Model file for the job. Use its own axes, mm. A direction names the side the tool comes from. Round coordinates to 2 decimals unless told otherwise and drop trailing zeros. Loops run counter-clockwise (first coordinate to the right, second up) from the corner with the lowest first, then second, coordinate; pieces in that order, holes last. Notation, with made-up numbers: (51.25, 43.25) -> (77.25, 43.25) arc R15 ccw to (77.25, 67.25) -> close; hole circle Ø5 at (22.25, 43.5). An arc over 180 degrees is marked (long way). Use a Markdown table: item, result. Add a question column.
```python
from build123d import *

# Parameters (mm, degrees)
SKETCH1_R           = 22.5
BOSS_EXTRUDE3_DEPTH = 20
SKETCH4_R           = 21
CUT_EXTRUDE2_DEPTH  = 10
SKETCH5_R           = 15
BOSS_EXTRUDE4_DEPTH = 20
SKETCH6_R           = 10
CUT_EXTRUDE4_DEPTH  = 20


with BuildPart() as part:
    # Sketch1 → Boss-Extrude3 (new body)
    with BuildSketch(Plane.XY):
        Circle(SKETCH1_R)
    extrude(amount=BOSS_EXTRUDE3_DEPTH)

    # Sketch4 → Cut-Extrude2 (cut)
    with BuildSketch(Plane.XY.offset(20)):
        Circle(SKETCH4_R)
    extrude(amount=-CUT_EXTRUDE2_DEPTH, mode=Mode.SUBTRACT)

    # Sketch5 → Boss-Extrude4 (add)
    with BuildSketch(Plane(origin=(0, 0, 0), x_dir=(-1, 0, 0), z_dir=(0, 0, -1))):
        Circle(SKETCH5_R)
    extrude(amount=BOSS_EXTRUDE4_DEPTH)

    # Sketch6 → Cut-Extrude4 (cut)
    with BuildSketch(Plane(origin=(0, 0, -20), x_dir=(-1, 0, 0), z_dir=(0, 0, -1))):
        Circle(SKETCH6_R)
    extrude(amount=-CUT_EXTRUDE4_DEPTH, mode=Mode.SUBTRACT)


solid = part.part
```
1) Cut at C-C on y = 17.5. Write the cut outline in (x, z), and give its area (3 significant figures).
2) Tool access for faces 4 (the face through (10.382, -19.961, 9.86)), 5 (the face through (0, 0, 10)), 6 (the face through (2.17, -9.76, -10.14)): list every direction of +Z, -Z, +X, -X, +Y, -Y with a clear straight run to the whole face (end or side of a thin tool).
3) Pin check, flat tips, straight feed: pin 1 Ø1 at (x, z) = (2.5, 14.5) entering from +Y; pin 2 Ø12.5 at (x, y) = (6, 9) entering from +Z; pin 3 Ø18 at (x, y) = (0, 0) entering from -Z; pin 4 Ø1.5 at (y, z) = (17, -14) entering from -X. Stop position of each tip, or through.
4) Cut at A-A on y = 0. Write the cut outline in (x, z), and give its area (3 significant figures).
5) Wall check: probe 1 along Y at (x, z) = (0, 14); probe 2 along Y at (x, z) = (0, -11.5); probe 3 along Z at (x, y) = (2, -1). Give the ranges that are in metal, low to high. Write a range as from..to.
6) Pull direction X, two halves, no side cores. Call faces 1 (the face through (-3, -10, -20)), 2 (the face through (14.985, 0.66, -9.86)), 3 (the face through (20.03, 6.31, 15.07)): +X half, -X half, draft (parallel to the pull), parting line (faces both ways), or undercut.
7) Cut at B-B on x = 18.5. Write the cut outline in (y, z), and give its area (3 significant figures).
Established:
| question | item | result |
|---|---|---|
| 1 | outline | (-14.14, 0) -> (14.14, 0) -> (14.14, 20) -> (11.61, 20) -> (11.61, 10) -> (-11.61, 10) -> (-11.61, 20) -> (-14.14, 20) -> close |
| 1 | area | 334 mm^2 |
| 2 | face 4 | +Z, -Z |
| 2 | face 5 | +Z |
| 2 | face 6 | -Z |
| 3 | pin 1 | stops at y = 22.41 |
| 3 | pin 2 | stops at z = 10 |
| 3 | pin 3 | stops at z = 0 |
| 3 | pin 4 | passes through |
| 4 | outline | (-22.5, 0) -> (-15, 0) -> (-15, -20) -> (-10, -20) -> (-10, 0) -> (10, 0) -> (10, -20) -> (15, -20) -> (15, 0) -> (22.5, 0) -> (22.5, 20) -> (21, 20) -> (21, 10) -> (-21, 10) -> (-21, 20) -> (-22.5, 20) -> close |
| 4 | area | 680 mm^2 |
| 5 | probe 1 | y = -22.5..-21, 21..22.5 |
| 5 | probe 2 | y = -15..-10, 10..15 |
| 5 | probe 3 | z = 0..10 |
| 6 | face 1 | draft |
| 6 | face 2 | parting line |
| 6 | face 3 | undercut |
| 7 | outline | (-12.81, 0) -> (12.81, 0) -> (12.81, 20) -> (9.94, 20) -> (9.94, 10) -> (-9.94, 10) -> (-9.94, 20) -> (-12.81, 20) -> close |
| 7 | area | 314 mm^2 |
